The drawing under review shows one solid part. Ordinate dimensions are in mm from its lowest x, y, z. A direction names the side the tool comes from. Give positions to 0.01 mm unless a question says otherwise; leave off trailing zeros. Loops run counter-clockwise (first coordinate to the right, second up) from the corner with the lowest first, then second, coordinate; pieces in that order, holes last. Notation, with made-up numbers: M -35,36 L -12,36 A26 ccw -12,70 Z; hole C -23,1 d4. An arc over 180 degrees is marked long. Write item = value, one per line. Start each with the question number.
1. We need section C-C on x = 34. Give the boundary of the cut face in (y, z), then the cut area to 3 significant figures.
2. For pin 1 (3 mm diameter, centred on x = 37.5, y = 7, fed in from +Z); pin 2 (14.5 mm diameter, centred on x = 58, y = 25.5, fed in from +Z); pin 3 (5 mm diameter, centred on x = 30, z = 33.5, fed in from +Y), all flat-tipped, find the tip position at first contact; note any pin that passes through.
3. We need section B-B on z = 56. Give the boundary of the cut face in (x, y), then the cut area to 3 significant figures.
4. Draft analysis for pull direction Z (two halves, no side actions). For the marked faces 1, 2, 3 and 4, state which applies: pulls with the +Z half, pulls with the -Z half, needs draft (parallel to the pull), parting line crosses it, or undercut.
5. We need section A-A on y = 7.5. Give the boundary of the cut face in (x, z), then the cut area to 3 significant figures.
6. We need section D-D on z = 42. Give the boundary of the cut face in (x, y).
7. Wall thickness on line 1 along Z through (x, y) = (88, 1.6); line 2 along X through (y, z) = (0.8, 3); line 3 along Z through (x, y) = (70, 5.5): over which ranges is each line inside the solid? List them lowest first. Write a range as from..to.
8. For the marked faces 5, 6, 7, 8 and 9, list the 3-axis set-ups (+Z, -Z, +X, -X, +Y, -Y) from which the entire face can be reached by the end or side of a thin tool; tool diameter is ignored.
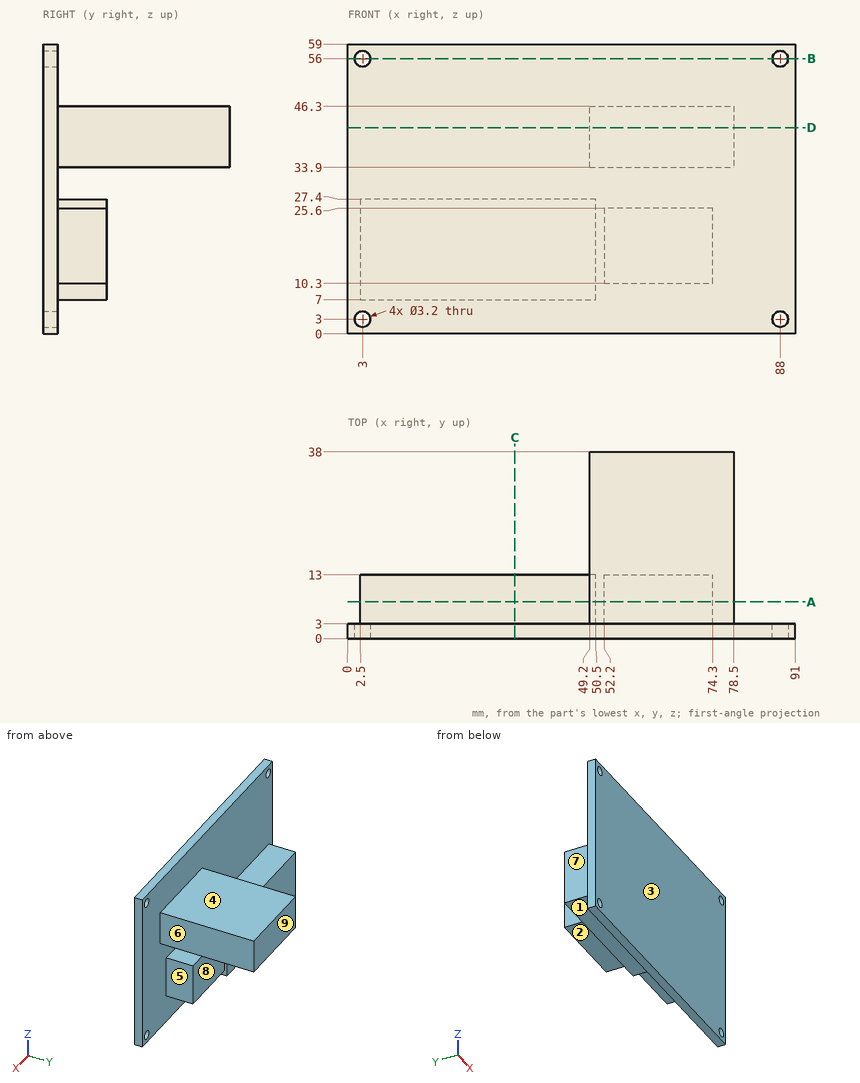
Final values:
q1.outline = M 0,0 L 3,0 L 3,7 L 13,7 L 13,27.4 L 3,27.4 L 3,59 L 0,59 Z
q1.area = 381 mm²
q2.pin_1 = 27.4
q2.pin_2 = 46.3
q2.pin_3 = 3
q3.outline = M 0,0 L 1.4,0 L 1.4,3 L 0,3 Z; M 4.6,0 L 86.4,0 L 86.4,3 L 4.6,3 Z; M 89.6,0 L 91,0 L 91,3 L 89.6,3 Z
q3.area = 254 mm²
q4.face_1 = pulls with the -Z half
q4.face_2 = undercut
q4.face_3 = needs draft
q4.face_4 = pulls with the +Z half
q5.outline = M 2.5,7 L 50.5,7 L 50.5,27.4 L 2.5,27.4 Z; M 49.2,33.9 L 78.5,33.9 L 78.5,46.3 L 49.2,46.3 Z; M 52.2,10.3 L 74.3,10.3 L 74.3,25.6 L 52.2,25.6 Z
q5.area = 1,680 mm²
q6.outline = M 0,0 L 91,0 L 91,3 L 78.5,3 L 78.5,38 L 49.2,38 L 49.2,3 L 0,3 Z
q7.line_1 = 0..1.4, 4.6..54.4, 57.6..59
q7.line_2 = 0..1.4, 4.6..86.4, 89.6..91
q7.line_3 = 10.3..25.6, 33.9..46.3
q8.face_5 = -Z, +X, +Y
q8.face_6 = +Z, -Z, +X, +Y
q8.face_7 = +Z, -Z, -X, +Y
q8.face_8 = -Z, +X, -X, +Y
q8.face_9 = +Z, -Z, +X, -X, +Y
